Could you check a few things on this model? Use its own coordinates, in mm. Give positions to 0.01 mm unless a question says otherwise; leave off trailing zeros. Order: outer loops, then holes, each group sorted by start corner. A loop starts at its lowest first (then second) coordinate and runs counter-clockwise, first axis right, second up.
(1) If I drill on probe 1 along Y at (x, z) = (0, 1.85); probe 2 along X at (y, z) = (-8.25, 2.9); probe 3 along X at (y, z) = (7.75, 4.4), over which ranges is the centre line in solid material (lowest first)?
(2) Imagine slicing it at D-D, the plane x = 7. Write out the boundary of the cut face in (y, z), then the cut area to 3 significant figures.
(3) Will these pins go through, and if not, where does the flat tip stop? pin 1 (2 mm diameter, centred on x = 7.78, y = -7.78, fed in from -Z); pin 2 (3 mm diameter, centred on x = 5, z = 1, fed in from +Y); pin 3 (2 mm diameter, centred on y = -3.5, z = 3.5, fed in from +X).
(4) Imagine slicing it at A-A, the plane y = 0. Write out the boundary of the cut face in (x, z), then the cut area to 3 significant figures.
(5) If we mould it in two halves opening along Y, with no side actions, what happens to faces 1 (the flat face through (6, 0, 0)), 2 (the cylindrical face through (12.524, 0.632, 2.958)), 3 (the cylindrical face through (-1.796, -13.683, 2.958))? For each: released by +Y, released by -Y, zero draft, split by the parting line, or undercut.
(6) Imagine slicing it at C-C, the plane y = 8.5. Write out the boundary of the cut face in (x, z).
Autodesk Inventor part; units mm, degrees
ref_plane "YZ Plane" through (0, 0, 0) normal (1, 0, 0) x (0, 1, 0)
ref_plane "XZ Plane" through (0, 0, 0) normal (0, 1, 0) x (-1, 0, 0)
ref_plane "XY Plane" through (0, 0, 0) normal (0, 0, 1) x (1, 0, 0)
ref_plane "작업 평면1" through (0, 0, 0) normal (0, 0, 1) x (1, 0, 0)
sketch "스케치1" plane through (0, 0, 0) normal (0, 0, 1) x (1, 0, 0)
  circle A0 centre (-7.778175, -7.778175) radius 1.55
  circle A1 centre (7.778175, -7.778175) radius 1.55
  circle A2 centre (7.778175, 7.778175) radius 1.55
  circle A3 centre (-7.778175, 7.778175) radius 1.55
  circle A4 centre (0, 0) radius 5
  circle A5 centre (0, 0) radius 13.9
  circle A6 centre (0, 11) radius 1.55
  circle A7 centre (11, 0) radius 1.55
  circle A8 centre (0, -11) radius 1.55
  circle A9 centre (-11, 0) radius 1.55
  circle A10 centre (-11, 0) radius 1.65
  circle A11 centre (-7.778175, 7.778175) radius 1.65
  circle A12 centre (0, 11) radius 1.65
  circle A13 centre (7.778175, 7.778175) radius 1.65
  circle A14 centre (11, 0) radius 1.65
  circle A15 centre (7.778175, -7.778175) radius 1.65
  circle A16 centre (0, -11) radius 1.65
  circle A17 centre (-7.778175, -7.778175) radius 1.65
  circle A18 centre (0, 0) radius 5.1
  circle A19 centre (0, 0) radius 13.8
  point P0 (0, 0)
  dimension "d0" = 0.1
  dimension "d1" = 0.1
  dimension "d2" = 0.1
  dimension "d3" = 0.1
  dimension "d4" = 0.1
  dimension "d5" = 0.1
  dimension "d6" = 0.1
  dimension "d7" = 0.1
  dimension "d8" = 0.1
  dimension "d9" = 0.1
sketch "스케치1 outline for 돌출1" plane through (0, 0, 0) normal (0, 0, 1) x (1, 0, 0)
  circle A0 centre (0, 0) radius 13.8
  circle A1 centre (-7.778175, -7.778175) radius 1.65
  circle A2 centre (-11, 0) radius 1.65
  circle A3 centre (0, -11) radius 1.65
  circle A4 centre (7.778175, -7.778175) radius 1.65
  circle A5 centre (0, 0) radius 5.1
  circle A6 centre (11, 0) radius 1.65
  circle A7 centre (-7.778175, 7.778175) radius 1.65
  circle A8 centre (0, 11) radius 1.65
  circle A9 centre (7.778175, 7.778175) radius 1.65
extrude "돌출1" add sketch "스케치1 outline for 돌출1" along normal blind 6
properties part number "25" material "아크릴, 선명"
Answer block:
1. probe 1: y = -13.8 to -12.65, -9.35 to -5.1, 5.1 to 9.35, 12.65 to 13.8
1. probe 2: x = -11.06 to -9.36, -6.2 to 6.2, 9.36 to 11.06
1. probe 3: x = -11.42 to -9.43, -6.13 to 6.13, 9.43 to 11.42
2. outline: (-11.89, 0) - (-9.23, 0) - (-9.23, 6) - (-11.89, 6) - close; (-6.32, 0) - (6.32, 0) - (6.32, 6) - (-6.32, 6) - close; (9.23, 0) - (11.89, 0) - (11.89, 6) - (9.23, 6) - close
2. area: 108 mm2
3. pin 1: passes through
3. pin 2: stops at y = 13.35
3. pin 3: stops at x = 13.57
4. outline: (-13.8, 0) - (-12.65, 0) - (-12.65, 6) - (-13.8, 6) - close; (-9.35, 0) - (-5.1, 0) - (-5.1, 6) - (-9.35, 6) - close; (5.1, 0) - (9.35, 0) - (9.35, 6) - (5.1, 6) - close; (12.65, 0) - (13.8, 0) - (13.8, 6) - (12.65, 6) - close
4. area: 64.8 mm2
5. face 1: zero draft
5. face 2: undercut
5. face 3: split by the parting line
6. outline: (-10.87, 0) - (-9.26, 0) - (-9.26, 6) - (-10.87, 6) - close; (-6.29, 0) - (6.29, 0) - (6.29, 6) - (-6.29, 6) - close; (9.26, 0) - (10.87, 0) - (10.87, 6) - (9.26, 6) - close
